Part model, mm, in its own coordinate system. Face numbers are marked on the shaded views. A direction names the side the tool comes from. Give positions to 0.01 mm unless a question says otherwise; leave off trailing zeros. Order: outer loops, then holes, each group sorted by start corner. A loop starts at its lowest first (then second) coordinate and runs counter-clockwise, first axis right, second up.
1. Slice it at C-C on y = -37. List the corners of the cut face in (x, z).
2. Slice it at D-D on y = -15. List the corners of the cut face in (x, z), and give its area (3 significant figures).
3. Slice it at A-A on y = -26.5. List the corners of the cut face in (x, z), and give its area (3 significant figures).
4. Mould opens along Y. For the marked faces 1, 2 and 3 say: +Y half, -Y half, draft (parallel to the pull), parting line (faces both ways), or undercut.
5. Drop flat-ended pins along their axis: pin 1 Ø1 at (x, y) = (-3, 8.5) entering from +Z; pin 2 Ø2 at (x, z) = (-10, 11) entering from +Y; pin 3 Ø1.9 at (x, y) = (-18.5, -0.5) entering from +Z. Give the stop position or say it passes through.
6. Probe line 1 (Z direction, x = -12, y = 31); line 2 (Y direction, x = -2.5, z = 20); line 3 (Y direction, x = -26.25, z = 22). List the from-to ranges inside material, lowest first.
7. Which spindle directions (+Z, -Z, +X, -X, +Y, -Y) get a long thin tool onto all of the face, cutting with end or side? Do the marked faces 4, 5 and 6. Say none if no direction does.
8. Slice it at B-B on y = 10. List the corners of the cut face in (x, z), and give its area (3 significant figures).
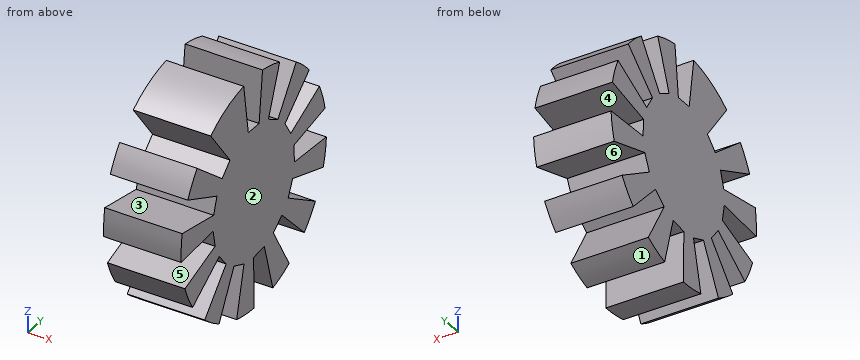
from build123d import *

# Parameters (mm, degrees)
F0_W            = 28.2793976367
F0_H            = 42.4683615565
F3_DEPTH        = 50.8
F3_COPIES_COUNT = 12
F3_COPIES_ANGLE = 316.8


# Not quite as in the source:
# - a feature of the source that left no trace in its solid (it failed there, or was rolled back) is left out
# - a pattern or mirror of a feature is missing from the dataset's text; its kind, count and spacing are read off the source's solid


with BuildPart() as f1:
    # F0 (on Front) → F1 (revolve)
    with BuildSketch(Plane.XZ):
        with Locations((-14.1396988183, 21.2341807783)):
            Rectangle(F0_W, F0_H)
    revolve(axis=Axis((-14.1396988183, 0, 0), (-1, 0, 0)))

    # F2 (on face) → F3 (cut)
    with BuildSketch(Plane(origin=(-28.2793976367, 0, 0), x_dir=(0, -1, 0), z_dir=(-1, 0, 0))):
        with BuildLine():
            ThreePointArc((5.8825213519, 42.0589785401), (0.3916223416, 42.4665558438), (-5.1058594535, 42.1603122917))
            Line((-5.1058594535, 42.1603122917), (-3.0962699093, 23.6033536494))
            Line((-3.0962699093, 23.6033536494), (0, 23.6033536494))
            Line((0, 23.6033536494), (3.2008844428, 23.6033536494))
            Line((3.2008844428, 23.6033536494), (5.8825213519, 42.0589785401))
        make_face()
    f3 = extrude(amount=-F3_DEPTH, mode=Mode.SUBTRACT)

    # F3_copies: F3 ×12 about axis
    f3_copies_axis = Axis((0, 0, 0), (-1, 0, 0))
    for i in range(1, F3_COPIES_COUNT):
        add(f3.rotate(f3_copies_axis, i * F3_COPIES_ANGLE / (F3_COPIES_COUNT - 1)), mode=Mode.SUBTRACT)


solid = f1.part
Data:
1. outline: (-28.28, -20.85) - (0, -20.85) - (0, -12.55) - (-28.28, -12.55) - close; (-28.28, -2.45) - (0, -2.45) - (0, 6.58) - (-28.28, 6.58) - close; (-28.28, 17.2) - (0, 17.2) - (0, 20.85) - (-28.28, 20.85) - close
2. outline: (-28.28, -27.32) - (0, -27.32) - (0, 18.29) - (-28.28, 18.29) - close; (-28.28, 20.78) - (0, 20.78) - (0, 39.73) - (-28.28, 39.73) - close
2. area: 1,830 mm2
3. outline: (-28.28, -33.19) - (0, -33.19) - (0, -28.96) - (-28.28, -28.96) - close; (-28.28, -16.84) - (0, -16.84) - (0, -8.92) - (-28.28, -8.92) - close; (-28.28, -1.6) - (0, -1.6) - (0, 4.77) - (-28.28, 4.77) - close; (-28.28, 12.49) - (0, 12.49) - (0, 21.39) - (-28.28, 21.39) - close
3. area: 776 mm2
4. face 1: +Y half
4. face 2: draft
4. face 3: undercut
5. pin 1: stops at z = 41.71
5. pin 2: stops at y = 41.27
5. pin 3: stops at z = 23.6
6. line 1: z = -29.03 to -19.54, -9.67 to -1.93, 6.28 to 14.67, 26.34 to 29.03
6. line 2: y = -37.46 to -24.75, -14.41 to 12.61, 14.65 to 23.63
6. line 3: y = -36.33 to -27.26, -15.92 to 8.98, 16.05 to 25.95
7. face 4: +X, -X, +Y
7. face 5: +X, -X, -Y
7. face 6: +X, -X
8. outline: (-28.28, -36.99) - (0, -36.99) - (0, 21.44) - (-28.28, 21.44) - close; (-28.28, 26.05) - (0, 26.05) - (0, 41.27) - (-28.28, 41.27) - close
8. area: 2,080 mm2
